Can you work these out from the model? Positions are in its coordinate system, mm. A direction names the side the tool comes from. Round coordinates to 2 decimals unless told otherwise and drop trailing zeros. Write each loop counter-clockwise with the first axis right and the second up, starting at its lowest first coordinate (ties: lowest second). Pieces come first, ordered by that corner, then holes. Notation, with made-up numbers: (58, -5.75) -> (91, -5.75) arc R21 ccw to (91, 25.25) -> close; hole circle Ø7 at (-31.5, -13). An arc over 180 degrees is marked (long way). Write item = value, one per line. Start each with the question number.
1) Imagine slicing it at A-A, the plane y = 4. State how many separate pieces and enclosed holes the cut face has, then the cut area to 3 significant figures.
2) Imagine slicing it at D-D, the plane x = 176.5. Please give me the cut outline in (y, z), then the cut area to 3 significant figures.
3) I'm going to push a flat-ended pin straight in: pin 1 (3 mm diameter, centred on x = 176.5, z = -10, fed in from +Y). Where does the tip first touch, or does it pass through?
4) If I drill on line 1 (X direction, y = 3.4, z = -51); line 2 (X direction, y = 0.95, z = -51); line 3 (Z direction, x = 68, y = 3.4), over which ranges is the centre line in solid material (lowest first)?
5) Thinking about a two-plate mould opening in Z: for faces 3 (the face through (180.99, 2.54, -58.15)), 4 (the face through (91, 5, -4)), 5 (the face through (157.236, 4.014, -30.715)), which applies, +Z half, -Z half, draft (parallel to the pull), parting line (faces both ways), or undercut?
6) For faces 1 (the face through (91, 3, -25)), 2 (the face through (2.85, 2.54, -3.01)), which set-ups out of +Z, -Z, +X, -X, +Y, -Y let a thin tool reach every point of the face, with its end or its side?
7) Imagine slicing it at B-B, the plane x = 92. Please give me the cut outline in (y, z).
8) Imagine slicing it at C-C, the plane z = -30.5. Please give me the cut outline in (x, y), then the cut area to 3 significant figures.
from build123d import *

# Parameters (mm, degrees)
SKETCH2_W           = 184
SKETCH2_H           = 61
SKETCH2_R           = 2
BOSS_EXTRUDE1_DEPTH = 5
SKETCH3_W           = 154
SKETCH3_H           = 51
SKETCH3_R           = 1.65
CUT_EXTRUDE1_DEPTH  = 2
FILLET1_R           = 10


with BuildPart() as part:
    # Sketch2 → Boss-Extrude1 (new body)
    with BuildSketch(Plane(origin=(0, 0, 0), x_dir=(1, 0, 0), z_dir=(0, 1, 0))):
        with Locations((92, 30.5)):
            Rectangle(SKETCH2_W, SKETCH2_H)
        with Locations(Location((7.5, 10, 0), (0, 0, 270))):
            Circle(SKETCH2_R, mode=Mode.SUBTRACT)
        with Locations(Location((176.5, 10, 0), (0, 0, 90))):
            Circle(SKETCH2_R, mode=Mode.SUBTRACT)
        with Locations(Location((176.5, 51, 0), (0, 0, 270))):
            Circle(SKETCH2_R, mode=Mode.SUBTRACT)
        with Locations(Location((7.5, 51, 0), (0, 0, 90))):
            Circle(SKETCH2_R, mode=Mode.SUBTRACT)
    extrude(amount=BOSS_EXTRUDE1_DEPTH)

    # Sketch3 → Cut-Extrude1 (cut)
    with BuildSketch(Plane(origin=(0, 5, 0), x_dir=(1, 0, 0), z_dir=(0, 1, 0))):
        with Locations((92, 30.5)):
            Rectangle(SKETCH3_W, SKETCH3_H)
        with Locations(Location((92, 30.5, 0), (0, 0, 270))):
            Circle(SKETCH3_R, mode=Mode.SUBTRACT)
        with Locations(Location((28.4, 30.5, 0), (0, 0, 270))):
            Circle(SKETCH3_R, mode=Mode.SUBTRACT)
        with Locations(Location((155.6, 30.5, 0), (0, 0, 270))):
            Circle(SKETCH3_R, mode=Mode.SUBTRACT)
    extrude(amount=-CUT_EXTRUDE1_DEPTH, mode=Mode.SUBTRACT)

    # Fillet1
    fillet1_edges = [part.edges().sort_by_distance(p)[0] for p in [
        (0, 2.5, -61),
        (184, 2.5, -61),
        (184, 2.5, 0),
        (0, 2.5, 0),
    ]]
    fillet(fillet1_edges, radius=FILLET1_R)


solid = part.part
Reported:
q1.separate_pieces = 4
q1.enclosed_holes = 5
q1.area = 3,260 mm²
q2.outline = (0, -60.68) -> (5, -60.68) -> (5, -53) -> (0, -53) -> close; (0, -49) -> (5, -49) -> (5, -12) -> (0, -12) -> close; (0, -8) -> (5, -8) -> (5, -0.32) -> (0, -0.32) -> close
q2.area = 262 mm²
q3.pin_1 = through
q4.line_1 = 0 to 5.5, 9.5 to 15, 169 to 174.5, 178.5 to 184
q4.line_2 = 0 to 5.5, 9.5 to 174.5, 178.5 to 184
q4.line_3 = -61 to -56, -5 to 0
q5.face_3 = -Z half
q5.face_4 = draft
q5.face_5 = undercut
q6.face_1 = +Y
q6.face_2 = +Z, -X, +Y, -Y
q7.outline = (0, -61) -> (5, -61) -> (5, -56) -> (3, -56) -> (3, -32.15) -> (5, -32.15) -> (5, -28.85) -> (3, -28.85) -> (3, -5) -> (5, -5) -> (5, 0) -> (0, 0) -> close
q8.outline = (0, 0) -> (184, 0) -> (184, 5) -> (169, 5) -> (169, 3) -> (157.25, 3) -> (157.25, 5) -> (153.95, 5) -> (153.95, 3) -> (93.65, 3) -> (93.65, 5) -> (90.35, 5) -> (90.35, 3) -> (30.05, 3) -> (30.05, 5) -> (26.75, 5) -> (26.75, 3) -> (15, 3) -> (15, 5) -> (0, 5) -> close
q8.area = 632 mm²
